Build history of the part. All positions in model axes, mm. A direction names the side the tool comes from. Round coordinates to 2 decimals unless told otherwise and drop trailing zeros. Write each loop counter-clockwise with the first axis right and the second up, starting at its lowest first coordinate (ties: lowest second). Pieces come first, ordered by that corner, then holes. Notation, with made-up numbers: (74, -30) -> (97, -30) arc R22 cw to (97, -16) -> close; hole circle Ø11 at (3, 56). An arc over 180 degrees is marked (long way). Answer in a Markdown table with one row per item.
```python
from build123d import *

# Parameters (mm, degrees)
SKETCH19_W                   = 215.9
SKETCH19_H                   = 76.2
BASE_FLANGE2_DEPTH           = 6.35
EDGE_FLANGE4_STRIP_W         = 38.1
EDGE_FLANGE4_STRIP_H         = 6.35
EDGE_FLANGE4_STRIP_CUT_DEPTH = 76.2
EDGE_FLANGE4_DEPTH           = 76.2
CUT_EXTRUDE1_REACH           = 240.78
SKETCH27_R                   = 7.14375


# Sheet-metal steps are written as plain solids
with BuildPart() as part:
    # Sketch19 → Base-Flange2 (new body)
    with BuildSketch(Plane.XY):
        Rectangle(SKETCH19_W, SKETCH19_H)
    extrude(amount=-BASE_FLANGE2_DEPTH)

    # Edge-Flange4 strip (across the edge) → Edge-Flange4 strip cut (cut)
    with BuildSketch(Plane(origin=(-107.95, 38.1, 0), x_dir=(1, 0, 0), z_dir=(0, -1, 0))):
        with Locations((-6.35, -3.175)):
            Rectangle(EDGE_FLANGE4_STRIP_W, EDGE_FLANGE4_STRIP_H)
    extrude(amount=EDGE_FLANGE4_STRIP_CUT_DEPTH, mode=Mode.SUBTRACT)

    # Edge-Flange4 section (across the edge) → Edge-Flange4 (add)
    with BuildSketch(Plane(origin=(-107.95, 38.1, 0), x_dir=(1, 0, 0), z_dir=(0, -1, 0))):
        with BuildLine():
            Line((0, 6.35), (0, 107.95))
            Line((0, 107.95), (6.35, 107.95))
            Line((6.35, 107.95), (6.35, 6.35))
            ThreePointArc((6.35, 6.35), (8.209871939, 1.859871939), (12.7, 0))
            Line((12.7, 0), (12.7, -6.35))
            ThreePointArc((12.7, -6.35), (3.719743879, -2.630256121), (0, 6.35))
        make_face()
    extrude(amount=EDGE_FLANGE4_DEPTH)

    # Sketch27 → Cut-Extrude1 (cut, up to next)
    with BuildSketch(Plane(origin=(-101.6, 0, 0), x_dir=(0, 0, -1), z_dir=(1, 0, 0)), mode=Mode.PRIVATE) as cut_extrude1_sk1:
        with Locations((-50.8, 0)):
            Circle(SKETCH27_R)
    cut_extrude1_tool1 = extrude(cut_extrude1_sk1.sketch, amount=-CUT_EXTRUDE1_REACH, mode=Mode.PRIVATE) & part.part
    add(cut_extrude1_tool1.solids().sort_by_distance((-101.6, 0, 50.8))[0], mode=Mode.SUBTRACT)


solid = part.part
```
Q1. Saw through at A-A on y = 0. Write the cut outline in (x, z).
A:
| item | result |
|---|---|
| outline | (-107.95, 6.35) arc R12.7 ccw to (-95.25, -6.35) -> (107.95, -6.35) -> (107.95, 0) -> (-95.25, 0) arc R6.35 cw to (-101.6, 6.35) -> (-101.6, 43.66) -> (-107.95, 43.66) -> close; (-107.95, 57.94) -> (-101.6, 57.94) -> (-101.6, 107.95) -> (-107.95, 107.95) -> close |
Q2. Saw through at D-D on x = -74. Write the cut outline in (y, z).
A:
| item | result |
|---|---|
| outline | (-38.1, -6.35) -> (38.1, -6.35) -> (38.1, 0) -> (-38.1, 0) -> close |
Q3. Drop a flat-ended pin along its axis: P1, Ø1.5, axis at x = -71, y = 2.5, coming from the +Z side. Give the stop position or say it passes through.
A:
| item | result |
|---|---|
| P1 | z = 0 |
Q4. Saw through at B-B on z = 50.8. Write the cut outline in (x, y), plus the area to 3 significant figures.
A:
| item | result |
|---|---|
| outline | (-107.95, -38.1) -> (-101.6, -38.1) -> (-101.6, -7.14) -> (-107.95, -7.14) -> close; (-107.95, 7.14) -> (-101.6, 7.14) -> (-101.6, 38.1) -> (-107.95, 38.1) -> close |
| area | 393 mm² |
Q5. Wall check: line 1 (Y direction, x = -103.75, z = 50.8); line 2 (X direction, y = -15.5, z = 73); line 3 (Z direction, x = -17.5, y = -8). Give the ranges that are in metal, low to high. Write a range as [from, to].
A:
| item | result |
|---|---|
| line 1 | [-38.1, -7.14], [7.14, 38.1] |
| line 2 | [-107.95, -101.6] |
| line 3 | [-6.35, 0] |
Q6. Which spindle directions (+Z, -Z, +X, -X, +Y, -Y) get a long thin tool onto all of the face, cutting with end or side? Do faces 1 (the flat face through (-107.95, 9, 56)), 2 (the flat face through (-101.6, 9, 58)). Say none if no direction does.
A:
| item | result |
|---|---|
| face 1 | +Z, -Z, -X, +Y, -Y |
| face 2 | +Z, +X, +Y, -Y |
Q7. Saw through at C-C on y = 20.5. Write the cut outline in (x, z), plus the area to 3 significant figures.
A:
| item | result |
|---|---|
| outline | (-107.95, 6.35) arc R12.7 ccw to (-95.25, -6.35) -> (107.95, -6.35) -> (107.95, 0) -> (-95.25, 0) arc R6.35 cw to (-101.6, 6.35) -> (-101.6, 107.95) -> (-107.95, 107.95) -> close |
| area | 2,030 mm² |
Q8. Two-plate mould, pull along Y, no slides. Class faces 3 (the cylindrical face through (-104.731, 0.314, 57.937)), 4 (the flat face through (-47, 38.1, -4)), 5 (the flat face through (5, 1, 0)), 6 (the flat face through (-47, -38.1, -4)): released by +Y, released by -Y, zero draft, split by the parting line, or undercut.
A:
| item | result |
|---|---|
| face 3 | undercut |
| face 4 | released by +Y |
| face 5 | zero draft |
| face 6 | released by -Y |
